Verification items for the finished model (mm, model axes). A direction names the side the tool comes from. Round coordinates to 2 decimals unless told otherwise and drop trailing zeros. Write each loop counter-clockwise with the first axis right and the second up, starting at its lowest first coordinate (ties: lowest second). Pieces come first, ordered by that corner, then holes. Notation, with made-up numbers: M 47,36 L 56,36 A23 ccw 56,51 Z; hole C -26.75,80.25 d3. An arc over 180 degrees is marked long. Answer in a Markdown table with one row per item. Add a question column.
1. Material ranges on probe 1 along Y at (x, z) = (8.5, 7.5); probe 2 along Y at (x, z) = (4, 2.1); probe 3 along Z at (x, y) = (9.75, 7.5), recorded low to high.
2. Draft check along Y on faces 3 (the flat face through (5, 0, 7)), 4 (the cylindrical face through (0.6, 22.43, 6.06)), 5 (the flat face through (0, 10.1, 3.6)). Enter one of: pulls with the +Y half, pulls with the -Y half, needs draft (parallel to the pull), parting line crosses it, or undercut.
3. Sectioned sample at A-A on x = 4. Record the cut outline in (y, z), plus the area to 3 significant figures.
4. Sectioned sample at D-D on x = 8.5. Record the cut outline in (y, z), plus the area to 3 significant figures.
5. Sectioned sample at C-C on z = 7.25. Record the cut outline in (x, y), plus the area to 3 significant figures.
6. Go/stop test with flat-tipped pins: pin 1 Ø3 at (y, z) = (7.5, 7) entering from -X; pin 2 Ø1 at (y, z) = (3, 9) entering from +X; pin 3 Ø4.5 at (x, y) = (4, 10) entering from +Z. Record where each tip stops, or that it passes through.
7. Set-up check for faces 1 (the flat face through (5, 20, 7)), 2 (the cylindrical face through (12.43, 22.4, 5.04)): record each of +Z, -Z, +X, -X, +Y, -Y from which the full face is reachable in a straight line by a thin tool's end or side.
Autodesk Inventor part; units mm, degrees
ref_plane "YZ Plane" through (0, 0, 0) normal (1, 0, 0) x (0, 1, 0)
ref_plane "XZ Plane" through (0, 0, 0) normal (0, 1, 0) x (-1, 0, 0)
ref_plane "XY Plane" through (0, 0, 0) normal (0, 0, 1) x (1, 0, 0)
sketch "Эскиз1" plane through (0, 0, 0) normal (0, 0, 1) x (1, 0, 0)
  line L0 (0, 0) -> (10, 0)
  line L1 (10, 0) -> (10, 20)
  line L2 (10, 20) -> (0, 20)
  line L3 (0, 20) -> (0, 0)
  circle A0 centre (4, 10) radius 2
  point P0 (10, 10)
  dimension "d0" = 10
  dimension "d1" = 4
  dimension "d2" = 6
  dimension "d3" = 20
extrude "Выдавливание1" add sketch "Эскиз1" along normal blind 4
sketch "Эскиз2" plane through (0, 0, 4) normal (0, 0, 1) x (1, 0, 0)
  point P0 (0, 0)
sketch "Эскиз3" plane through (0, 0, 0) normal (0, 0, 1) x (1, 0, 0)
  line L0 (0, 23) -> (13, 23)
  line L1 (13, 23) -> (13, -3)
  line L2 (13, -3) -> (0, -3)
  line L3 (0, -3) -> (0, 23)
  line L4 (10, 0) -> (10, 20)
  line L5 (10, 20) -> (0, 20)
  line L6 (0, 0) -> (10, 0)
  point P0 (10, 10)
  point P1 (13, 10)
  dimension "d8" = 3
  dimension "d10" = 3
extrude "Выдавливание2" add sketch "Эскиз3" along normal blind 10 contours L0 L1 L2 L3 L6 L4 L5
fillet "Сопряжение1" radius 2 11 edges at (13, 10, 0) (6.5, -3, 0) (6.5, 23, 0) (0, 10, 0) (13, 23, 5) (13, 10, 10) (13, -3, 5) (6.5, -3, 10) (6.5, 23, 10) (0, 23, 5) (0, -3, 5)
properties part number "2"
Geometry check:
| question | item | result |
|---|---|---|
| 1 | probe 1 | y = -3 to 0, 20 to 23 |
| 1 | probe 2 | y = -3 to 8, 12 to 23 |
| 1 | probe 3 | z = 0 to 4 |
| 2 | face 3 | undercut |
| 2 | face 4 | pulls with the +Y half |
| 2 | face 5 | needs draft |
| 3 | outline | M -3,2 A2 ccw -1,0 L 8,0 L 8,4 L 0,4 L 0,10 L -1,10 A2 ccw -3,8 Z; M 12,0 L 21,0 A2 ccw 23,2 L 23,8 A2 ccw 21,10 L 20,10 L 20,4 L 12,4 Z |
| 3 | area | 121 mm2 |
| 4 | outline | M -3,2 A2 ccw -1,0 L 21,0 A2 ccw 23,2 L 23,8 A2 ccw 21,10 L 20,10 L 20,4 L 0,4 L 0,10 L -1,10 A2 ccw -3,8 Z |
| 4 | area | 137 mm2 |
| 5 | outline | M 0,-1 A2 ccw 2,-3 L 11,-3 A2 ccw 13,-1 L 13,21 A2 ccw 11,23 L 2,23 A2 ccw 0,21 L 0,20 L 10,20 L 10,0 L 0,0 Z |
| 5 | area | 135 mm2 |
| 6 | pin 1 | stops at x = 10 |
| 6 | pin 2 | stops at x = 12.94 |
| 6 | pin 3 | stops at z = 4 |
| 7 | face 1 | +Z, -X |
| 7 | face 2 | +Z, -Z, +X, +Y |
